from build123d import *

# Parameters (mm, degrees)
SKETCH021_R           = 42.45
SKETCH021_R_2         = 0.75
SKETCH021_W           = 23.5
SKETCH021_H           = 12.8
PAD010_DEPTH          = 17.5
SKETCH025_R           = 1
POCKET013_DEPTH       = 5
POLARPATTERN002_COUNT = 3
POLARPATTERN002_ANGLE = 180


with BuildPart() as part:
    # Sketch021 → Pad010 (new body)
    with BuildSketch(Plane.XY):
        Circle(SKETCH021_R)
        with Locations((8.25, 0)):
            Circle(SKETCH021_R_2, mode=Mode.SUBTRACT)
        with Locations((-20.05, 0)):
            Circle(SKETCH021_R_2, mode=Mode.SUBTRACT)
        with BuildLine():
            ThreePointArc((6.249999, -10.825318), (12.5, -2e-06), (6.250002, 10.825316))
            Line((4.071802, 23.052558), (6.250002, 10.825316))
            Line((17.475007, 30.267584), (4.071802, 23.052558))
            ThreePointArc((17.474996, -30.26759), (34.95, -6e-06), (17.475007, 30.267584))
            Line((17.474996, -30.26759), (4.071794, -23.052559))
            Line((6.249999, -10.825318), (4.071794, -23.052559))
        make_face(mode=Mode.SUBTRACT)
        with Locations((-5.9, 0)):
            Rectangle(SKETCH021_W, SKETCH021_H, mode=Mode.SUBTRACT)
    extrude(amount=PAD010_DEPTH)

    # Sketch025 (on DatumPlane) → Pocket013 (cut)
    with BuildSketch(Plane.YZ.offset(42.45)):
        with Locations((0, 8.75)):
            Circle(SKETCH025_R)
    pocket013 = extrude(amount=-POCKET013_DEPTH, mode=Mode.SUBTRACT)

    # PolarPattern002: Pocket013 ×3 about axis
    polarpattern002_axis = Axis((0, 0, 0), (0, 0, 1))
    for i in range(1, POLARPATTERN002_COUNT):
        add(pocket013.rotate(polarpattern002_axis, i * POLARPATTERN002_ANGLE / (POLARPATTERN002_COUNT - 1)), mode=Mode.SUBTRACT)


solid = part.part
Verification items for the finished model (mm, model axes). A direction names the side the tool comes from. Round coordinates to 2 decimals unless told otherwise and drop trailing zeros. Write each loop counter-clockwise with the first axis right and the second up, starting at its lowest first coordinate (ties: lowest second). Pieces come first, ordered by that corner, then holes.
(1) Mould release check, pull along Y, two halves, no side actions. Record for faces 5 (the cylindrical face through (34.946, -0.512, 8.628)), 6 (the cylindrical face through (-5.53, 42.09, 8.63)), 7 (the flat face through (-10, -9, 0)): pulls with the +Y half, pulls with the -Y half, needs draft (parallel to the pull), parting line crosses it, or undercut.
Returned:
face 5: undercut
face 6: parting line crosses it
face 7: needs draft
(2) Access from +Z, -Z, +X, -X, +Y, -Y to the whole of each face (thin tool, end or side, straight path). Record for faces 1 (the flat face through (-37.45, 0, 9)), 2 (the cylindrical face through (39.98, -0.13, 9.74)), 3 (the cylindrical face through (0.13, 39.99, 9.74)), 4 (the flat face through (-17.65, 0, 9)).
Returned:
face 1: -X
face 2: +X
face 3: +Y
face 4: +Z, -Z
(3) Material ranges on line 1 (Z direction, x = 0, y = 38); line 2 (X direction, y = 4, z = 12.5); line 3 (Y direction, x = 8.25, z = 13.25), recorded low to high.
Returned:
line 1: z = 0 to 7.75, 9.75 to 17.5
line 2: x = -42.26 to -17.65, 5.85 to 11.84, 34.72 to 42.26
line 3: y = -41.64 to -25.3, -9.39 to -0.75, 0.75 to 9.39, 25.3 to 41.64
(4) Section check C-C (y = -14). Enter the section's corners in (x, z).
Returned:
outline: (-40.07, 0) - (5.68, 0) - (5.68, 17.5) - (-40.07, 17.5) - close; (32.02, 0) - (40.07, 0) - (40.07, 17.5) - (32.02, 17.5) - close
(5) Section check B-B (x = 0). Enter the section's corners in (y, z), plus the area to 3 significant figures.
Returned:
outline: (-42.45, 0) - (-6.4, 0) - (-6.4, 17.5) - (-42.45, 17.5) - close; (6.4, 0) - (42.45, 0) - (42.45, 7.75) - (37.45, 7.75) - (37.45, 9.75) - (42.45, 9.75) - (42.45, 17.5) - (6.4, 17.5) - close
area: 1,250 mm2
(6) Depth check by flat-ended pin: pin 1 Ø2 at (y, z) = (0.5, 9) entering from -X; pin 2 Ø3 at (x, z) = (-5.5, 4.5) entering from +Y; pin 3 Ø1.2 at (y, z) = (0, 8.75) entering from -X; pin 4 Ø0.6 at (y, z) = (-0.5, 8.5) entering from +X. Enter the tip coordinate at first touch or a pass-through.
Returned:
pin 1: stops at x = -42.45
pin 2: stops at y = 42.26
pin 3: stops at x = -37.45
pin 4: stops at x = 37.45
(7) Section check A-A (z = 12.25). Enter the section's corners in (x, y) (3 decimals), plus the area to 3 significant figures.
Returned:
outline: circle Ø84.9 at (0, 0); hole circle Ø1.5 at (-20.05, 0); hole (-17.65, -6.4) - (5.85, -6.4) - (5.85, 6.4) - (-17.65, 6.4) - close; hole (4.072, -23.053) - (17.475, -30.268) arc R34.95 ccw to (17.475, 30.268) - (4.072, 23.053) - (6.25, 10.825) arc R12.5 cw to (6.25, -10.825) - close; hole circle Ø1.5 at (8.25, 0)
area: 4,060 mm2
(8) Section check D-D (x = -15). Enter the section's corners in (y, z).
Returned:
outline: (-39.71, 0) - (-6.4, 0) - (-6.4, 17.5) - (-39.71, 17.5) - close; (6.4, 0) - (39.71, 0) - (39.71, 17.5) - (6.4, 17.5) - close
